Verification items for the finished model (mm, model axes). Give positions to 0.01 mm unless a question says otherwise; leave off trailing zeros. Write each loop counter-clockwise with the first axis right and the second up, starting at its lowest first coordinate (ties: lowest second). Pieces come first, ordered by that corner, then holes. Notation, with made-up numbers: (32, 33.5) -> (42, 33.5) arc R23 ccw to (42, 45.5) -> close; hole circle Ø10 at (21.5, -14.75). An arc over 180 degrees is marked (long way). Use one line per item in the form item = value. Start each with the question number.
(1) Section check A-A, the plane x = -25. Record the cut outline in (y, z).
(2) Depth check by flat-ended pin: pin 1 Ø0.8 at (x, z) = (-1.5, -176) entering from +Y; pin 2 Ø1.4 at (x, z) = (-1, -531.5) entering from -Y; pin 3 Ø3 at (x, z) = (-1.5, -276) entering from +Y. Enter the tip coordinate at first touch or a pass-through.
(3) Scan lines: L1, parallel to X at y = 16, z = -685; L2, parallel to Y at x = -22, z = -236; L3, parallel to X at y = 15, z = -195 (3 decimals). Record each from-to range of solid material in increasing order.
(4) Section check B-B, the plane y = 0. State how many separate pieces and enclosed holes the cut face has, plus the area to 3 significant figures.
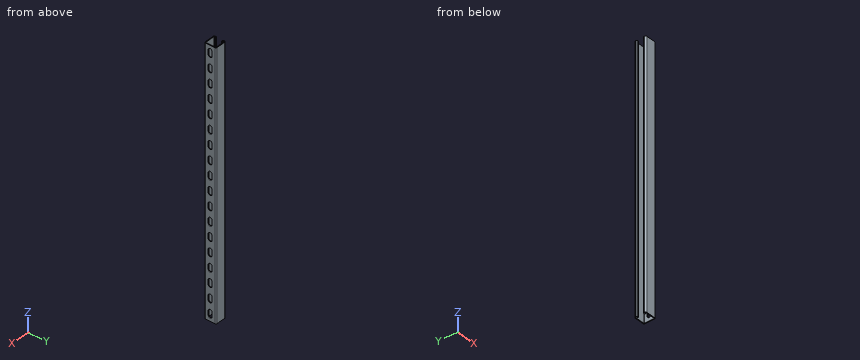
from build123d import *

# Parameters (mm, degrees)
BOSS_EXTRUDE1_DEPTH = 914.4
CUT_EXTRUDE1_DEPTH  = 2.794
LPATTERN1_COUNT     = 18
LPATTERN1_PITCH     = 50.8


with BuildPart() as part:
    # Sketch1 → Boss-Extrude1 (new body)
    with BuildSketch(Plane.XY):
        with BuildLine():
            Line((-36.22675, 20.6375), (-3.46075, 20.6375))
            ThreePointArc((-3.46075, 20.6375), (-1.013630207, 19.623869793), (0, 17.17675))
            Line((0, 17.17675), (0, -17.17675))
            ThreePointArc((0, -17.17675), (-1.013630207, -19.623869793), (-3.46075, -20.6375))
            Line((-3.46075, -20.6375), (-36.22675, -20.6375))
            ThreePointArc((-36.22675, -20.6375), (-39.796401808, -19.158901808), (-41.275, -15.58925))
            Line((-41.275, -15.58925), (-41.275, -14.57325))
            ThreePointArc((-41.275, -14.57325), (-40.261369793, -12.126130207), (-37.81425, -11.1125))
            Line((-37.81425, -11.1125), (-35.5346, -11.1125))
            ThreePointArc((-35.5346, -11.1125), (-34.1376, -12.5095), (-35.5346, -13.9065))
            Line((-35.5346, -13.9065), (-37.81425, -13.9065))
            ThreePointArc((-37.81425, -13.9065), (-38.285713446, -14.101786554), (-38.481, -14.57325))
            Line((-38.481, -14.57325), (-38.481, -15.58925))
            ThreePointArc((-38.481, -15.58925), (-37.820745461, -17.183245461), (-36.22675, -17.8435))
            Line((-36.22675, -17.8435), (-3.46075, -17.8435))
            ThreePointArc((-3.46075, -17.8435), (-2.989286554, -17.648213446), (-2.794, -17.17675))
            Line((-2.794, -17.17675), (-2.794, 17.17675))
            ThreePointArc((-2.794, 17.17675), (-2.989286554, 17.648213446), (-3.46075, 17.8435))
            Line((-3.46075, 17.8435), (-36.22675, 17.8435))
            ThreePointArc((-36.22675, 17.8435), (-37.820745461, 17.183245461), (-38.481, 15.58925))
            Line((-38.481, 15.58925), (-38.481, 14.57325))
            ThreePointArc((-38.481, 14.57325), (-38.285713446, 14.101786554), (-37.81425, 13.9065))
            Line((-37.81425, 13.9065), (-35.5346, 13.9065))
            ThreePointArc((-35.5346, 13.9065), (-34.1376, 12.5095), (-35.5346, 11.1125))
            Line((-35.5346, 11.1125), (-37.81425, 11.1125))
            ThreePointArc((-37.81425, 11.1125), (-40.261369793, 12.126130207), (-41.275, 14.57325))
            Line((-41.275, 14.57325), (-41.275, 15.58925))
            ThreePointArc((-41.275, 15.58925), (-39.796401808, 19.158901808), (-36.22675, 20.6375))
        make_face()
    extrude(amount=-BOSS_EXTRUDE1_DEPTH)

    # Sketch2 → Cut-Extrude1 (cut)
    with BuildSketch(Plane(origin=(0, 0, 0), x_dir=(0, 0, -1), z_dir=(1, 0, 0))):
        with BuildLine():
            Line((18.25625, 7.14375), (32.54375, 7.14375))
            ThreePointArc((32.54375, 7.14375), (39.6875, 0), (32.54375, -7.14375))
            Line((32.54375, -7.14375), (18.25625, -7.14375))
            ThreePointArc((18.25625, -7.14375), (11.1125, 0), (18.25625, 7.14375))
        make_face()
    cut_extrude1 = extrude(amount=-CUT_EXTRUDE1_DEPTH, mode=Mode.SUBTRACT)

    # LPattern1: Cut-Extrude1 ×18
    with Locations(*[(0, 0, -i * LPATTERN1_PITCH) for i in range(1, LPATTERN1_COUNT)]):
        add(cut_extrude1, mode=Mode.SUBTRACT)


solid = part.part
Completed:
q1.outline = (-20.64, -914.4) -> (-17.84, -914.4) -> (-17.84, 0) -> (-20.64, 0) -> close; (17.84, -914.4) -> (20.64, -914.4) -> (20.64, 0) -> (17.84, 0) -> close
q2.pin_1 = 20.27
q2.pin_2 = -20.16
q2.pin_3 = 20.61
q3.L1 = -41.26 to -38.44, -2.79 to 0
q3.L2 = -20.64 to -17.84, 17.84 to 20.64
q3.L3 = -41.275 to -38.481, -2.794 to 0
q4.separate_pieces = 19
q4.enclosed_holes = 0
q4.area = 1,120 mm²
